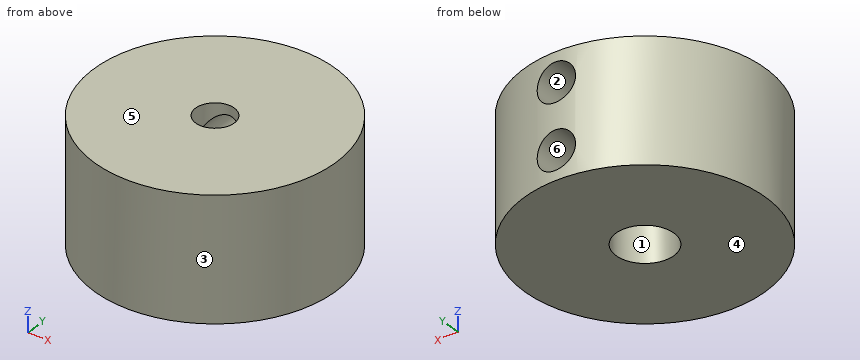
Autodesk Inventor part; units mm, degrees
ref_plane "YZ Plane" through (0, 0, 0) normal (1, 0, 0) x (0, 1, 0)
ref_plane "XZ Plane" through (0, 0, 0) normal (0, 1, 0) x (-1, 0, 0)
ref_plane "XY Plane" through (0, 0, 0) normal (0, 0, 1) x (1, 0, 0)
sketch "Sketch1" plane through (0, 0, 0) normal (0, 0, 1) x (1, 0, 0)
  circle A0 centre (0, 0) radius 12.5
  circle A1 centre (0, 0) radius 2
  dimension "d1" = 4
  dimension "d32" = 25
extrude "Extrusion1" add sketch "Sketch1" along normal blind 12.7
sketch "Sketch8" plane through (0, 0, 0) normal (0, 1, 0) x (-1, 0, 0)
  circle A0 centre (0, 3) radius 2
  circle A1 centre (0, 9.7) radius 2
  line L0 (2, 0) -> (-2, 0)
  line L1 (-2, 12.7) -> (2, 12.7)
  point P0 (0, 0)
  point P1 (0, 0)
  dimension "d33" = 4
  dimension "d34" = 4
  dimension "d35" = 3
  dimension "d36" = 3
extrude "Extrusion6" cut sketch "Sketch8" along normal through all
sketch "Sketch9" plane through (0, 0, 0) normal (0, 0, -1) x (-1, 0, 0)
  circle A0 centre (0, 0) radius 3
  dimension "d39" = 6
extrude "Extrusion7" cut sketch "Sketch9" against normal blind 6.35
thread "Thread1"
thread "Thread2"
properties part number "AA050" material "Aluminum 6061"
Input: part model. Units: mm. Frame: model coordinates. Face numbers are marked on the shaded views. A direction names the side the tool comes from. Give positions to 0.01 mm unless a question says otherwise; leave off trailing zeros. Order: outer loops, then holes, each group sorted by start corner. A loop starts at its lowest first (then second) coordinate and runs counter-clockwise, first axis right, second up. Notation, with made-up numbers: (58.5, 67.25) - (78.5, 67.25) arc R20 ccw to (78.5, 94.25) - close; hole circle Ø9 at (-0.5, 15.5). An arc over 180 degrees is marked (long way). Use a Markdown table: item, result.
(1) Section query C-C (y = -7.5). Output: boundary loops of the cut face in (x, z).
Computed values:
| item | result |
|---|---|
| outline | (-10, 0) - (10, 0) - (10, 12.7) - (-10, 12.7) - close |
(2) Access query for the marked faces 1, 2 and 3. Directions: +Z, -Z, +X, -X, +Y, -Y. A direction counts if a zero-diameter tool reaches every point of the face in a straight line with its end or side. Return the directions, or none.
Computed values:
| item | result |
|---|---|
| face 1 | -Z |
| face 2 | +Y |
| face 3 | +Z, -Z |
(3) Section query B-B (y = -0.5). Output: boundary loops of the cut face in (x, z), then the cut area to 3 significant figures.
Computed values:
| item | result |
|---|---|
| outline | (-12.49, 0) - (-2.96, 0) - (-2.96, 6.35) - (-1.94, 6.35) - (-1.94, 12.7) - (-12.49, 12.7) - close; (1.94, 6.35) - (2.96, 6.35) - (2.96, 0) - (12.49, 0) - (12.49, 12.7) - (1.94, 12.7) - close |
| area | 255 mm2 |
(4) Draft query along Z for the marked faces 4, 5 and 6. Return one class per face: released by +Z, released by -Z, zero draft, split by the parting line, or undercut.
Computed values:
| item | result |
|---|---|
| face 4 | released by -Z |
| face 5 | released by +Z |
| face 6 | undercut |
(5) Pin query (flat end, axial travel): pin 1 (8 mm diameter, centred on x = 0, y = 0, fed in from +Z); pin 2 (1 mm diameter, centred on y = 5.5, z = 10.5, fed in from +X); pin 3 (1.5 mm diameter, centred on y = 1.5, z = 6, fed in from -X); pin 4 (2 mm diameter, centred on y = 1.5, z = 4.5, fed in from +X). Return the tip coordinate at first contact, or that it passes through.
Computed values:
| item | result |
|---|---|
| pin 1 | stops at z = 12.7 |
| pin 2 | stops at x = 11.46 |
| pin 3 | stops at x = -12.48 |
| pin 4 | stops at x = 12.49 |
(6) Section query A-A (x = 0). Output: boundary loops of the cut face in (y, z), then the cut area to 3 significant figures.
Computed values:
| item | result |
|---|---|
| outline | (-12.5, 0) - (-3, 0) - (-3, 6.35) - (-2, 6.35) - (-2, 12.7) - (-12.5, 12.7) - close; (2, 6.35) - (3, 6.35) - (3, 5) - (12.5, 5) - (12.5, 7.7) - (2, 7.7) - close; (2, 11.7) - (12.5, 11.7) - (12.5, 12.7) - (2, 12.7) - close; (3, 0) - (12.5, 0) - (12.5, 1) - (3, 1) - close |
| area | 174 mm2 |
(7) Section query D-D (y = 6.25). Output: boundary loops of the cut face in (x, z).
Computed values:
| item | result |
|---|---|
| outline | (-10.83, 0) - (10.83, 0) - (10.83, 12.7) - (-10.83, 12.7) - close; hole circle Ø4 at (0, 3); hole circle Ø4 at (0, 9.7) |
(8) Line query: line 1 (X direction, y = 9.5, z = 8.5); line 2 (Y direction, x = 0, z = 9); line 3 (X direction, y = 7.25, z = 3). Output: solid intervals per line, ascending. Write a range as from..to.
Computed values:
| item | result |
|---|---|
| line 1 | x = -8.12..-1.6, 1.6..8.12 |
| line 2 | y = -12.5..-2 |
| line 3 | x = -10.18..-2, 2..10.18 |
